Geometry: final body of the model. Coordinates: model frame, mm. A direction names the side the tool comes from. Round coordinates to 2 decimals unless told otherwise and drop trailing zeros. Loops run counter-clockwise (first coordinate to the right, second up) from the corner with the lowest first, then second, coordinate; pieces in that order, holes last. Notation, with made-up numbers: M 87,-16.5 L 122,-16.5 A5 ccw 122,-10.5 Z; hole C -16,25 d3. An arc over 180 degrees is marked long. Answer as a JSON object with one key per item and string values.
from build123d import *

# Parameters (mm, degrees)
F1_DEPTH = 15.5448
F2_R     = 15.452898
F3_W     = 221.588438
F3_H     = 121.92
F4_DEPTH = 12.192


with BuildPart() as f1:
    # F0 (on Top) → F1 (new body)
    with BuildSketch(Plane.XY):
        with BuildLine():
            ThreePointArc((0, 36.634617), (-18.317308, 18.317308), (0, 0))
            Line((0, 0), (44.156924, 0))
            ThreePointArc((44.156924, 0), (62.474232, 18.317308), (44.156924, 36.634617))
            Line((44.156924, 36.634617), (0, 36.634617))
        make_face()
    extrude(amount=F1_DEPTH)

    # F2
    f2_edges = [f1.edges().sort_by_distance(p)[0] for p in [
        (22.078462, 36.634617, 0),
        (62.474232, 18.317308, 0),
        (-18.317308, 18.317308, 0),
    ]]
    fillet(f2_edges, radius=F2_R)


with BuildPart() as f4:
    # F3 (on Top) → F4 (new body)
    with BuildSketch(Plane.XY):
        with Locations((25.399999, 10.16)):
            Rectangle(F3_W, F3_H)
    extrude(amount=F4_DEPTH)

    # F5: cut F1
    add(f1.part, mode=Mode.SUBTRACT)


with BuildPart() as f4_1:
    # F6: moved
    add(f4.part.moved(Location((0, 0, -2.7432))))


solid = f4_1.part
1) Section query A-A (x = 7). Return the cut outline in (y, z).
Results:
{"outline": "M -50.8,-2.74 L 15.45,-2.74 A15.45 cw 0.35,9.45 L -50.8,9.45 Z; M 21.18,-2.74 L 71.12,-2.74 L 71.12,9.45 L 36.29,9.45 A15.45 cw Z"}
2) Ray query, line 1 (Y direction, x = 6, z = 3); line 2 (Y direction, x = 8.5, z = 2.75); line 3 (X direction, y = 24, z = 8.75). Return the intervals inside material, ascending.
Results:
{"line 1": "-50.8 to 3.43, 33.2 to 71.12", "line 2": "-50.8 to 3.64, 33 to 71.12", "line 3": "-85.39 to -16.87, 61.03 to 136.19"}
3) Reachability of faces 4 (the cylindrical face through (22.39, 5.63, 0.78)), 5 (the flat face through (-85.394, 9, 3)) from +Z, -Z, +X, -X, +Y, -Y: full face, straight path, thin tool, end or side. Return the list, or none.
Results:
{"face 4": "+Z", "face 5": "+Z, -Z, -X, +Y, -Y"}
4) Pull-direction query (Y, two-part tool) for faces 1 (the cylindrical face through (21.769, 31.001, 0.778)), 2 (the flat face through (136.194, 9, 3)), 3 (the flat face through (24, 71.12, 3)); classes: +Y half, -Y half, draft (parallel to the pull), parting line (faces both ways), or undercut.
Results:
{"face 1": "undercut", "face 2": "draft", "face 3": "+Y half"}
